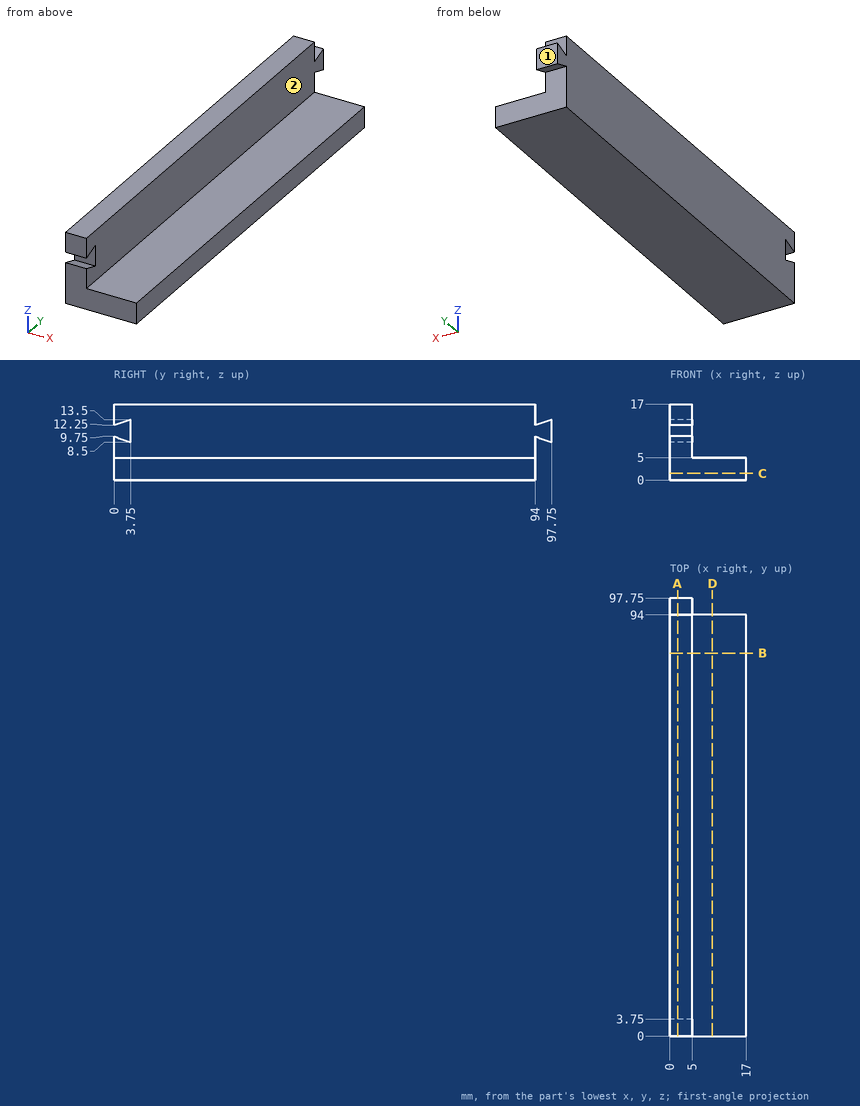
Check sheet for the drawn part. Datum: minimum x, y, z corner. Units: mm. A direction names the side the tool comes from. Round coordinates to 2 decimals unless told otherwise and drop trailing zeros. Order: outer loops, then holes, each group sorted by start corner. A loop starts at its lowest first (then second) coordinate and runs counter-clockwise, first axis right, second up. Notation, with made-up numbers: M 14.25,-21.5 L 66.25,-21.5 A16 ccw 66.25,-3.5 Z; hole C -35.5,76 d11. An arc over 180 degrees is marked long. Answer in a Markdown table with one row per item.
(1) Section check D-D on x = 9.5. Record the boundary of the cut face in (y, z).
Findings:
| item | result |
|---|---|
| outline | M 0,0 L 94,0 L 94,5 L 0,5 Z |
(2) Set-up check for the marked faces 1 and 2: record each of +Z, -Z, +X, -X, +Y, -Y from which the full face is reachable in a straight line by a thin tool's end or side.
Findings:
| item | result |
|---|---|
| face 1 | +Z, -Z, +X, -X, +Y |
| face 2 | +Z, +X, +Y, -Y |
(3) Section check B-B on y = 85.5. Record the boundary of the cut face in (x, z).
Findings:
| item | result |
|---|---|
| outline | M 0,0 L 17,0 L 17,5 L 5,5 L 5,17 L 0,17 Z |
(4) Section check A-A on x = 1.75. Record the boundary of the cut face in (y, z).
Findings:
| item | result |
|---|---|
| outline | M 0,0 L 94,0 L 94,9.75 L 97.75,8.5 L 97.75,13.5 L 94,12.25 L 94,17 L 0,17 L 0,12.25 L 3.75,13.5 L 3.75,8.5 L 0,9.75 Z |
(5) Gauge pin test, flat ends, axial feed: pin 1 (3 mm diameter, centred on x = 6, z = 4, fed in from +Y); pin 2 (6 mm diameter, centred on x = 13, y = 48, fed in from +Z); pin 3 (3.5 mm diameter, centred on y = 42.5, z = 12, fed in from +X). Record the tip position at first contact, or that the pin passes through.
Findings:
| item | result |
|---|---|
| pin 1 | stops at y = 94 |
| pin 2 | stops at z = 5 |
| pin 3 | stops at x = 5 |
(6) Material ranges on line 1 along Z through (x, y) = (11.25, 17); line 2 along Y through (x, z) = (1, 1.5), recorded low to high. Write a range as from..to.
Findings:
| item | result |
|---|---|
| line 1 | z = 0..5 |
| line 2 | y = 0..94 |
(7) Section check C-C on z = 1.5. Record the boundary of the cut face in (x, y).
Findings:
| item | result |
|---|---|
| outline | M 0,0 L 17,0 L 17,94 L 0,94 Z |
